from build123d import *

# Parameters (mm, degrees)
F0_W     = 38.1
F0_H     = 50.8
F1_DEPTH = 3.175
F2_SIZE  = 1.27
F4_D     = 1.27


with BuildPart() as f1:
    # F0 (on Front) → F1 (new body)
    with BuildSketch(Plane.XZ):
        Rectangle(F0_W, F0_H)
    extrude(amount=F1_DEPTH)

    # F2
    f2_edges = [f1.edges().sort_by_distance(p)[0] for p in [
        (19.05, -3.175, 0),
        (0, -3.175, 25.4),
        (-19.05, -3.175, 0),
        (0, -3.175, -25.4),
    ]]
    chamfer(f2_edges, length=F2_SIZE)

    # F4 (through all)
    with Locations(Plane.XZ.offset(3.175)):
        with Locations((-14.610798, 8.786894), (3.81, -19.063698), (14.610798, -4.976894), (-14.610798, 4.976894), (3.81, 19.063698), (14.610798, -8.786894), (-3.81, 19.063698), (-14.610798, -8.786894), (14.610798, 4.976894), (14.610798, 8.786894), (-14.610798, -4.976894), (-3.81, -19.063698)):
            Hole(F4_D / 2)


solid = f1.part
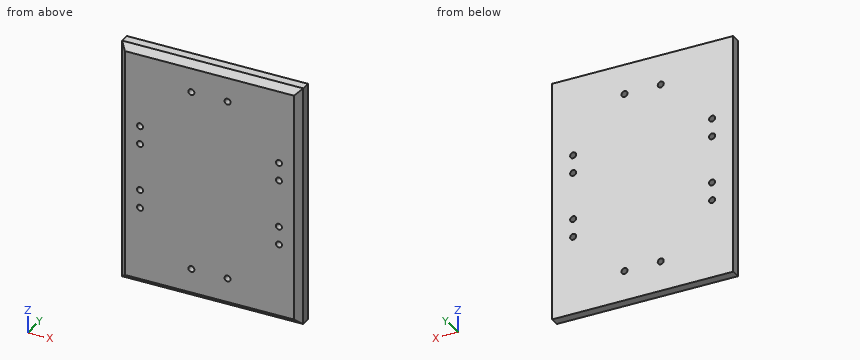
Could you check a few things on this model? Use its own coordinates, in mm. Give positions to 0.01 mm unless a question says otherwise; leave off trailing zeros. Loops run counter-clockwise (first coordinate to the right, second up) from the corner with the lowest first, then second, coordinate; pieces in that order, holes last. Notation, with made-up numbers: (1.25, -8.5) -> (41.25, -8.5) arc R23 ccw to (41.25, 24.5) -> close; hole circle Ø3 at (71, -2). An arc over 180 degrees is marked (long way). Return JSON: item names as keys, results as strings.
Item 1: If we section it at B-B on y = -2.65: Count the separate pieces of the cut face and the enclosed holes in it, plus the area to 3 significant figures.
Geometry results:
{"separate pieces": "1", "enclosed holes": "12", "area": "1,790 mm²"}
Item 2: If we section it at A-A on x = 3.81: List the corners of the cut face in (y, z) for me (3 decimals).
Geometry results:
{"outline": "(-3.175, -24.13) -> (-1.905, -25.4) -> (0, -25.4) -> (0, -19.699) -> (-3.175, -19.699) -> close; (-3.175, -18.429) -> (0, -18.429) -> (0, 18.429) -> (-3.175, 18.429) -> close; (-3.175, 19.699) -> (0, 19.699) -> (0, 25.4) -> (-1.905, 25.4) -> (-3.175, 24.13) -> close"}
Item 3: I need wall thicknesses on L1, parallel to Z at x = -3.81, y = -1.2; L2, parallel to X at y = -1.6, z = -5.5; L3, parallel to X at y = -0.3, z = 8.5. Which ranges of each line are inside material? Lowest first, please. Write a range as from..to.
Geometry results:
{"L1": "z = -25.4..-19.7, -18.43..18.43, 19.7..25.4", "L2": "x = -19.05..-14.97, -14.25..14.25, 14.97..19.05", "L3": "x = -19.05..-15.18, -14.04..14.04, 15.18..19.05"}
Item 4: I'm going to push a flat-ended pin straight in: pin 1 (1.1 mm diameter, centred on x = 14.61, z = -8.79, fed in from -Y). Where does the tip first touch, or does it pass through?
Geometry results:
{"pin 1": "passes through"}
